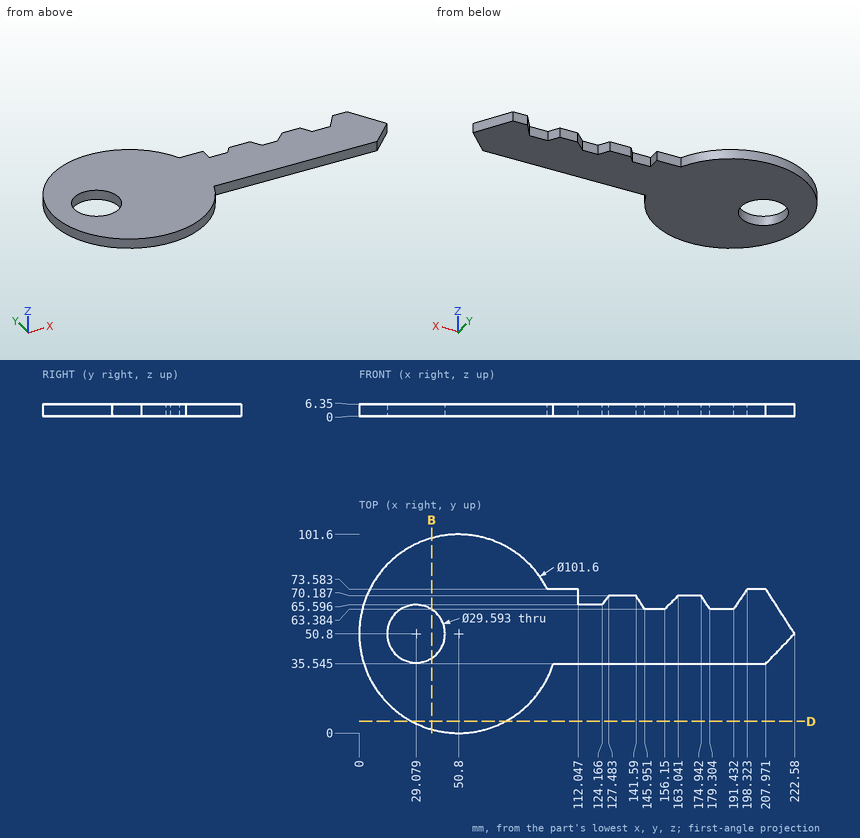
Answer from the drawing. Dimensions are ordinates in mm from the lowest x, y and z of the part. Give positions to 0.01 mm unless a question says otherwise; leave off trailing zeros. Order: outer loops, then holes, each group sorted by start corner. A loop starts at its lowest first (then second) coordinate and runs counter-clockwise, first axis right, second up. Notation, with made-up numbers: (26.25, -12) - (64.25, -12) arc R18 ccw to (64.25, 19) - close; hole circle Ø6 at (11.25, 65). An arc over 180 degrees is marked (long way). One line per item, written item: value. Start each with the question number.
1. Consider line 1 (X direction, y = 50.8, z = 4.75) (1 decimal); line 2 (X direction, y = 57, z = 4.25) (1 decimal); line 3 (Y direction, x = 155, z = 1.5) (1 decimal). Determine where each line is inside the solid, lowest interval first.
2. Section B-B, the plane x = 37 is taken. Write down the section's boundary in (y, z), then the cut area to 3 significant figures.
3. Each of these flat-tipped pins is pushed along its axis until it touches: pin 1 Ø3 at (x, z) = (131.5, 3.5) entering from +Y; pin 2 Ø1.9 at (x, z) = (187.5, 3) entering from +Y; pin 3 Ø1.9 at (y, z) = (68, 2.5) entering from +X; pin 4 Ø2 at (x, z) = (51.5, 1.5) entering from -Y. Where does it stop, or does it pass through?
4. Section D-D, the plane y = 6 is taken. Write down the section's boundary in (x, z), then the cut area to 3 significant figures.
Filled sheet:
1. line 1: 0 to 14.3, 43.9 to 222.6
1. line 2: 0.4 to 15.6, 42.5 to 218.6
1. line 3: 35.5 to 63.4
2. outline: (1.91, 0) - (38.3, 0) - (38.3, 6.35) - (1.91, 6.35) - close; (63.3, 0) - (99.69, 0) - (99.69, 6.35) - (63.3, 6.35) - close
2. area: 462 mm²
3. pin 1: y = 70.19
3. pin 2: y = 63.38
3. pin 3: x = 212.16
3. pin 4: y = 0
4. outline: (26.85, 0) - (74.75, 0) - (74.75, 6.35) - (26.85, 6.35) - close
4. area: 304 mm²
